Work out the finished part from the listing and answer in its coordinate system (mm). A direction names the side the tool comes from. Coordinates: 2 decimals unless noted, no trailing zeros. Loops run counter-clockwise (first coordinate to the right, second up) from the corner with the lowest first, then second, coordinate; pieces in that order, holes last. Notation, with made-up numbers: (34.5, 60) -> (82.5, 60) arc R24 cw to (82.5, 96) -> close; hole circle Ø3 at (22.5, 15). An arc over 180 degrees is marked (long way). Use a Markdown table: item, result.
from build123d import *

# Parameters (mm, degrees)
BLOCOBASE_DEPTH           = 5
SKFIXACAO_R               = 1.7
SKFIXACAO_R_2             = 1.55
FIXACAO_DEPTH             = 5.15
RESSALTOFIXACAO_DEPTH     = 0.15
BOTAO_DEPTH               = 2.15
SKETCH5_W                 = 6.3
SKETCH5_H                 = 1
BASECONECTORNONC_DEPTH    = 10.5
SKDESENHOCONECTORNONC_R   = 0.75
DESENHOCONECTORNONC_DEPTH = 20.5
BASECONECTORCOM_DEPTH     = 3.15
SKDESENHOCONECTORCOM_R    = 0.75
DESENHOCONECTORCOM_DEPTH  = 1
BASECONTATO_DEPTH         = 3.15
SKAPOIOROLO_R             = 0.7
APOIOROLO_DEPTH           = 1
SKROLO_R                  = 2.5
ROLO_DEPTH                = 4.3
SKETCH6_W                 = 15.037683952
SKETCH6_H                 = 10.848275608
CUT_EXTRUDE1_DEPTH        = 10
SKETCH7_W                 = 6.3
SKETCH7_H                 = 1
BOSS_EXTRUDE1_DEPTH       = 0.001


with BuildPart() as part:
    # skBlocoBase → BlocoBase (new body, symmetric)
    with BuildSketch(Plane(origin=(0, 0, 0), x_dir=(0, 0, -1), z_dir=(1, 0, 0))):
        with BuildLine():
            Line((-10.7, 7.95), (10.7, 7.95))
            ThreePointArc((10.7, 7.95), (12.9627417, 7.0127417), (13.9, 4.75))
            Line((13.9, 4.75), (13.9, -4.75))
            ThreePointArc((13.9, -4.75), (12.9627417, -7.0127417), (10.7, -7.95))
            Line((10.7, -7.95), (-10.7, -7.95))
            ThreePointArc((-10.7, -7.95), (-12.9627417, -7.0127417), (-13.9, -4.75))
            Line((-13.9, -4.75), (-13.9, 4.75))
            ThreePointArc((-13.9, 4.75), (-12.9627417, 7.0127417), (-10.7, 7.95))
        make_face()
    extrude(amount=BLOCOBASE_DEPTH, both=True)

    # skFixacao → Fixacao (cut, symmetric)
    with BuildSketch(Plane(origin=(0, 0, 0), x_dir=(0, 0, -1), z_dir=(1, 0, 0))):
        with Locations((-11.125, -5.1)):
            Circle(SKFIXACAO_R)
        with Locations((11.125, 5.1)):
            Circle(SKFIXACAO_R_2)
    extrude(amount=FIXACAO_DEPTH, both=True, mode=Mode.SUBTRACT)

    # skRessaltoFixacao → RessaltoFixacao (add)
    with BuildSketch(Plane(origin=(5, 0, 0), x_dir=(0, 0, -1), z_dir=(1, 0, 0))):
        with BuildLine():
            ThreePointArc((-8.475, -5.525), (-9.353679656, -3.403679656), (-11.475, -2.525))
            Line((-11.475, -2.525), (-13.7, -2.525))
            Line((-13.7, -2.525), (-13.7, -4.75))
            ThreePointArc((-13.7, -4.75), (-12.821320344, -6.871320344), (-10.7, -7.75))
            Line((-10.7, -7.75), (-8.475, -7.75))
            Line((-8.475, -7.75), (-8.475, -5.525))
        make_face()
        with BuildLine():
            ThreePointArc((-9.789845005, -6.152312282), (-10.474438165, -6.670595205), (-11.325, -6.788194302))
            ThreePointArc((-11.325, -6.788194302), (-11.775561835, -3.529404795), (-9.789845005, -6.152312282))
        make_face(mode=Mode.SUBTRACT)
        with BuildLine():
            ThreePointArc((13.775, 4.675), (12.896320344, 6.796320344), (10.775, 7.675))
            Line((10.775, 7.675), (8.55, 7.675))
            Line((8.55, 7.675), (8.55, 5.45))
            ThreePointArc((8.55, 5.45), (9.428679656, 3.328679656), (11.55, 2.45))
            Line((11.55, 2.45), (13.775, 2.45))
            Line((13.775, 2.45), (13.775, 4.675))
        make_face()
        with BuildLine():
            ThreePointArc((12.353274612, 4.1545681), (11.71815932, 3.667986725), (10.925, 3.562957385))
            ThreePointArc((10.925, 3.562957385), (10.53184068, 6.532013275), (12.353274612, 4.1545681))
        make_face(mode=Mode.SUBTRACT)
    ressaltofixacao = extrude(amount=RESSALTOFIXACAO_DEPTH)

    # MirrorRessaltoFixacao: RessaltoFixacao across plane
    add(ressaltofixacao.mirror(Plane(origin=(0, 0, 0), x_dir=(0, 0, 1), z_dir=(1, 0, 0))))

    # skBotao → Botao (add, symmetric)
    with BuildSketch(Plane(origin=(0, 0, 0), x_dir=(0, 0, -1), z_dir=(1, 0, 0))):
        with BuildLine():
            Line((-10.475, 7.95), (-10.475, 8.6))
            ThreePointArc((-10.475, 8.6), (-9.075, 9.6), (-7.675, 8.6))
            Line((-7.675, 8.6), (-7.675, 7.95))
            Line((-7.675, 7.95), (-10.475, 7.95))
        make_face()
    extrude(amount=BOTAO_DEPTH, both=True)

    # Sketch5 → BaseConectorNONC (add)
    with BuildSketch(Plane(origin=(0, 0, -13.9), x_dir=(-1, 0, 0), z_dir=(0, 0, -1))):
        with Locations((0, -3.975)):
            Rectangle(SKETCH5_W, SKETCH5_H)
        with Locations((0, 3.975)):
            Rectangle(SKETCH5_W, SKETCH5_H)
    extrude(amount=BASECONECTORNONC_DEPTH)

    # skDesenhoConectorNONC → DesenhoConectorNONC (cut)
    with BuildSketch(Plane.XZ.offset(4.475)):
        Polygon((2.65, -22.767142952), (1.616967042, -24.4), (3.15, -24.4), (3.15, -18.161236833), (2.65, -18.161236833), align=None)
        Polygon((-3.15, -24.4), (-1.616967042, -24.4), (-2.65, -22.767142952), (-2.65, -18.161236833), (-3.15, -18.161236833), align=None)
        with Locations((0, -22.767142952)):
            Circle(SKDESENHOCONECTORNONC_R)
    extrude(amount=-DESENHOCONECTORNONC_DEPTH, mode=Mode.SUBTRACT)

    # skBaseConectorCOM → BaseConectorCOM (add, symmetric)
    with BuildSketch(Plane(origin=(0, 0, 0), x_dir=(0, 0, -1), z_dir=(1, 0, 0))):
        with BuildLine():
            Line((9.725, -11.25), (0.225, -11.25))
            ThreePointArc((0.225, -11.25), (-0.482106781, -10.957106781), (-0.775, -10.25))
            Line((-0.775, -10.25), (-0.775, -7.95))
            Line((-0.775, -7.95), (0.225, -7.95))
            Line((0.225, -7.95), (0.225, -9.25))
            ThreePointArc((0.225, -9.25), (0.517893219, -9.957106781), (1.225, -10.25))
            Line((1.225, -10.25), (9.725, -10.25))
            Line((9.725, -10.25), (9.725, -11.25))
        make_face()
    extrude(amount=BASECONECTORCOM_DEPTH, both=True)

    # skDesenhoConectorCOM → DesenhoConectorCOM (cut)
    with BuildSketch(Plane.XZ.offset(11.25)):
        Polygon((2.65, -8.092142952), (1.616967042, -9.725), (3.15, -9.725), (3.15, -3.486236833), (2.65, -3.486236833), align=None)
        Polygon((-3.15, -9.725), (-1.616967042, -9.725), (-2.65, -8.092142952), (-2.65, -3.486236833), (-3.15, -3.486236833), align=None)
        with Locations((0, -8.092142952)):
            Circle(SKDESENHOCONECTORCOM_R)
    extrude(amount=-DESENHOCONECTORCOM_DEPTH, mode=Mode.SUBTRACT)

    # skBaseContato → BaseContato (add, symmetric)
    with BuildSketch(Plane(origin=(0, 0, 0), x_dir=(0, 0, -1), z_dir=(1, 0, 0))):
        with BuildLine():
            Line((2.63302332, 7.95), (2.63302332, 8.486635004))
            ThreePointArc((2.63302332, 8.486635004), (2.497665983, 8.828739854), (2.164880406, 8.985619098))
            Line((2.164880406, 8.985619098), (-24.4, 10.681624431))
            Line((-24.4, 10.681624431), (-24.336285828, 11.679592619))
            Line((-24.336285828, 11.679592619), (3.545575005, 9.899506131))
            ThreePointArc((3.545575005, 9.899506131), (3.878360582, 9.742626887), (4.013717919, 9.400522037))
            Line((4.013717919, 9.400522037), (4.013717919, 7.95))
            Line((4.013717919, 7.95), (2.63302332, 7.95))
        make_face()
    extrude(amount=BASECONTATO_DEPTH, both=True)

    # skApoioRolo → ApoioRolo (add)
    with BuildSketch(Plane(origin=(3.15, 0, 0), x_dir=(0, 0, -1), z_dir=(1, 0, 0))):
        with BuildLine():
            ThreePointArc((-21.354211514, 14.486814776), (-22.754211514, 15.886814776), (-24.154211514, 14.486814776))
            Line((-24.154211514, 14.486814776), (-24.336285828, 11.679592619))
            Line((-24.336285828, 11.679592619), (-22.939130364, 11.590392778))
            Line((-22.939130364, 11.590392778), (-21.541974901, 11.501192936))
            Line((-21.541974901, 11.501192936), (-21.365242034, 14.3114187))
            Line((-21.365242034, 14.3114187), (-21.354211514, 14.486814776))
        make_face()
        with Locations((-22.754211514, 14.486814776)):
            Circle(SKAPOIOROLO_R, mode=Mode.SUBTRACT)
    apoiorolo = extrude(amount=-APOIOROLO_DEPTH)

    # MirrorApoioRolo: ApoioRolo across plane
    add(apoiorolo.mirror(Plane(origin=(0, 0, 0), x_dir=(0, 0, 1), z_dir=(1, 0, 0))))

    # skRolo → Rolo (add)
    with BuildSketch(Plane.ZY.offset(-2.15)):
        with Locations((22.754211514, 14.486814776)):
            Circle(SKROLO_R)
    extrude(amount=ROLO_DEPTH)

    # Sketch6 → Cut-Extrude1 (cut)
    with BuildSketch(Plane(origin=(0, 10.084763511, -0.643850544), x_dir=(1, 0, 0), z_dir=(0, 0.997968188, -0.063714172))):
        with Locations((-4.368841976, -23.671158356)):
            Rectangle(SKETCH6_W, SKETCH6_H)
    extrude(amount=CUT_EXTRUDE1_DEPTH, mode=Mode.SUBTRACT)

    # Sketch7 → Boss-Extrude1 (add)
    with BuildSketch(Plane(origin=(0, 1.594829108, 24.980136372), x_dir=(1, 0, 0), z_dir=(0, 0.063714172, 0.997968188))):
        with Locations((0, 9.605295572)):
            Rectangle(SKETCH7_W, SKETCH7_H)
    extrude(amount=BOSS_EXTRUDE1_DEPTH)


solid = part.part
Q1. Given pin 1 Ø5 at (x, z) = (-0.5, -19.5) entering from -Y (3 decimals); pin 2 Ø0.8 at (x, y) = (-0.5, -10.5) entering from -Z (3 decimals); pin 3 Ø5 at (x, z) = (-2.5, 17) entering from -Y, each flat-ended and moving along its own axis, determine where each tip first touches the part or whether it passes through.
Solved:
| item | result |
|---|---|
| pin 1 | y = -4.475 |
| pin 2 | z = -9.725 |
| pin 3 | y = 10.05 |
Q2. For faces 1 (the cylindrical face through (0.04, -9.95, -0.51)), 2 (the cylindrical face through (-0.163, -10.757, -8.824)), 3 (the flat face through (3.15, -10, 0)), 4 (the flat face through (-2.65, -11, -6)), determine the directions among +Z, -Z, +X, -X, +Y, -Y from which every point of the face is accessible in a straight line to the end or side of a thin tool.
Solved:
| item | result |
|---|---|
| face 1 | -Z, +X, -X |
| face 2 | -Y |
| face 3 | +Z, -Z, +X, -Y |
| face 4 | -Z, -X, -Y |
Q3. Section D-D on y = -1.5 is taken. Determine the outline of the cut face in (x, z), and give its area (3 significant figures).
Solved:
| item | result |
|---|---|
| outline | (-5, -13.9) -> (5, -13.9) -> (5, 13.9) -> (-5, 13.9) -> close |
| area | 278 mm² |
Q4. Consider line 1 (Y direction, x = -1.5, z = -14.5) (3 decimals); line 2 (Y direction, x = -1.5, z = -1); line 3 (Z direction, x = 0, y = -3.7). Determine where each line is inside the solid, lowest interval first. Write a range as [from, to].
Solved:
| item | result |
|---|---|
| line 1 | [-4.475, -3.475], [3.475, 4.475] |
| line 2 | [-11.25, -10.22], [-7.95, 7.95], [9.06, 10.06] |
| line 3 | [-24.4, -23.52], [-22.02, 10.16], [12.09, 13.9] |
Q5. Section A-A on x = 4.25 is taken. Determine the outline of the cut face in (y, z) (3 decimals).
Solved:
| item | result |
|---|---|
| outline | (-7.95, -10.7) arc R3.2 ccw to (-4.75, -13.9) -> (4.75, -13.9) arc R3.2 ccw to (7.95, -10.7) -> (7.95, 10.7) arc R3.2 ccw to (4.75, 13.9) -> (-4.75, 13.9) arc R3.2 ccw to (-7.95, 10.7) -> close; hole circle Ø3.4 at (-5.1, 11.125); hole circle Ø3.1 at (5.1, -11.125) |
Q6. Determine the mould class of faces 5 (the flat face through (0, -3.475, -18)), 6 (the cylindrical face through (0.07, -6.988, -12.987)), 7 (the flat face through (-5, 0, 0)) for opening direction Y: pulls with the +Y half, pulls with the -Y half, needs draft (parallel to the pull), parting line crosses it, or undercut.
Solved:
| item | result |
|---|---|
| face 5 | undercut |
| face 6 | pulls with the -Y half |
| face 7 | needs draft |
Q7. Section C-C on x = 0 is taken. State how many separate pieces and enclosed holes the cut face has, and give its area (3 significant figures).
Solved:
| item | result |
|---|---|
| separate pieces | 4 |
| enclosed holes | 2 |
| area | 480 mm² |
Q8. Section B-B on z = 2 is taken. Determine the outline of the cut face in (x, y).
Solved:
| item | result |
|---|---|
| outline | (-5, -7.95) -> (5, -7.95) -> (5, 7.95) -> (-5, 7.95) -> close; (-3.15, 9.25) -> (3.15, 9.25) -> (3.15, 10.25) -> (-3.15, 10.25) -> close |
